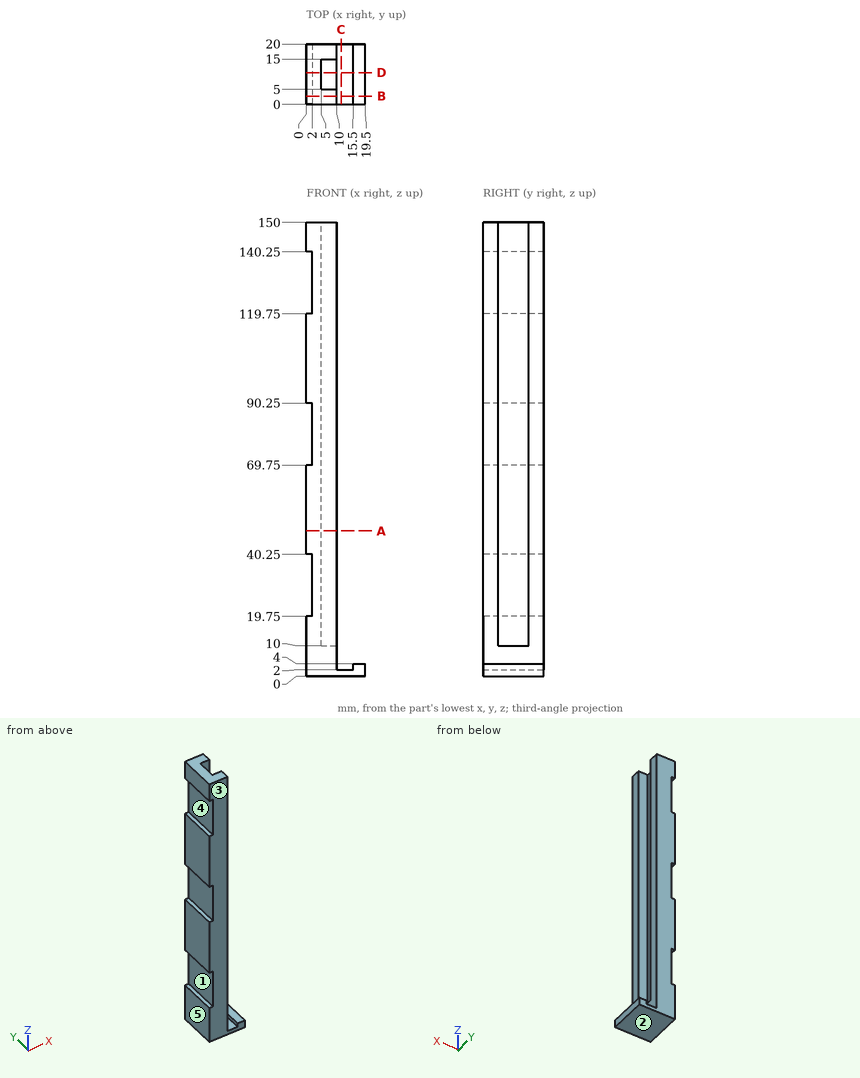
Input: dimensioned drawing with shaded views. Units: mm. Origin: part minimum x, y, z. A direction names the side the tool comes from. Coordinates: 2 decimals unless noted, no trailing zeros. Order: outer loops, then holes, each group sorted by start corner. A loop starts at its lowest first (then second) coordinate and runs counter-clockwise, first axis right, second up.
(1) Draft query along Z for the marked faces 1, 2 and 3. Return one class per face: pulls with the +Z half, pulls with the -Z half, needs draft (parallel to the pull), parting line crosses it, or undercut.
(2) Access query for the marked faces 4 and 5. Directions: +Z, -Z, +X, -X, +Y, -Y. A direction counts if a zero-diameter tool reaches every point of the face in a straight line with its end or side. Return the directions, or none.
(3) Section query C-C (x = 11.5). Return the cut outline in (y, z), plus the area to 3 significant figures.
(4) Material intervals for probe 1 along Y at (x, z) = (8.5, 65); probe 2 along X at (y, z) = (1, 37.5); probe 3 along Z at (x, y) = (13.25, 3), sorted ascending.
(5) First-contact query: pin 1 (2 mm diameter, centred on x = 18, y = 11.5, fed in from +Z); pin 2 (2 mm diameter, centred on y = 5, z = 125, fed in from +X). Flat tips, straight axial feed; report the tip coordinate or a pass-through.
(6) Section query A-A (z = 48). Return the cut outline in (x, y), plus the area to 3 significant figures.
(7) Section query D-D (y = 10.5). Return the cut outline in (x, z), plus the area to 3 significant figures.
(8) Section query B-B (y = 2.75). Return the cut outline in (x, z).
Solution:
1. face 1: undercut
1. face 2: pulls with the -Z half
1. face 3: needs draft
2. face 4: -X, +Y, -Y
2. face 5: +Z, -Z, -X, +Y, -Y
3. outline: (0, 0) - (20, 0) - (20, 2) - (0, 2) - close
3. area: 40.0 mm2
4. probe 1: y = 0 to 5, 15 to 20
4. probe 2: x = 2 to 10
4. probe 3: z = 0 to 2
5. pin 1: stops at z = 4
5. pin 2: stops at x = 10
6. outline: (0, 0) - (10, 0) - (10, 5) - (5, 5) - (5, 15) - (10, 15) - (10, 20) - (0, 20) - close
6. area: 150 mm2
7. outline: (0, 0) - (19.5, 0) - (19.5, 4) - (15.5, 4) - (15.5, 2) - (10, 2) - (10, 10) - (5, 10) - (5, 150) - (0, 150) - (0, 140.25) - (2, 140.25) - (2, 119.75) - (0, 119.75) - (0, 90.25) - (2, 90.25) - (2, 69.75) - (0, 69.75) - (0, 40.25) - (2, 40.25) - (2, 19.75) - (0, 19.75) - close
7. area: 704 mm2
8. outline: (0, 0) - (19.5, 0) - (19.5, 4) - (15.5, 4) - (15.5, 2) - (10, 2) - (10, 150) - (0, 150) - (0, 140.25) - (2, 140.25) - (2, 119.75) - (0, 119.75) - (0, 90.25) - (2, 90.25) - (2, 69.75) - (0, 69.75) - (0, 40.25) - (2, 40.25) - (2, 19.75) - (0, 19.75) - close
